Design review of the part built by this model. Coordinates are the model's own, in mm. Face numbers are marked on the shaded views. A direction names the side the tool comes from. Coordinates: 2 decimals unless noted, no trailing zeros. Loops run counter-clockwise (first coordinate to the right, second up) from the corner with the lowest first, then second, coordinate; pieces in that order, holes last. Notation, with made-up numbers: M 14.5,15.25 L 67.5,15.25 A12 ccw 67.5,19.25 Z; hole C -23,57 d6. An arc over 180 degrees is marked long. Put each result on its own line as item: value. Start each with the question number.
(1) For probe 1 along X at (y, z) = (35.25, 2.75); probe 2 along X at (y, z) = (-35.25, 5.75), list the stretches that pass through material, from the lowest coordinate up. Write a range as [from, to].
(2) Take a section at C-C, the plane y = 0. Give the boundary of the cut face in (x, z).
(3) For the marked faces 4, 5 and 6, list the 3-axis set-ups (+Z, -Z, +X, -X, +Y, -Y) from which the entire face can be reached by the end or side of a thin tool; tool diameter is ignored.
(4) Take a section at B-B, the plane x = -1. Give the boundary of the cut face in (y, z), then the cut area to 3 significant figures.
(5) Clearance check with a flat-ended pin moving along its axis: pin 1 (3.5 mm diameter, centred on x = -6.5, y = 31, fed in from +Z). State where the tip first meets the part, or that it passes through.
(6) Take a section at D-D, the plane y = 35.25. Give the boundary of the cut face in (x, z), then the cut area to 3 significant figures.
(7) The part is to be moulded in two halves that separate along X. For the marked faces 1, 2 and 3, say which applies: +X half, -X half, draft (parallel to the pull), parting line (faces both ways), or undercut.
(8) Take a section at A-A, the plane y = 14.5. Give the boundary of the cut face in (x, z).
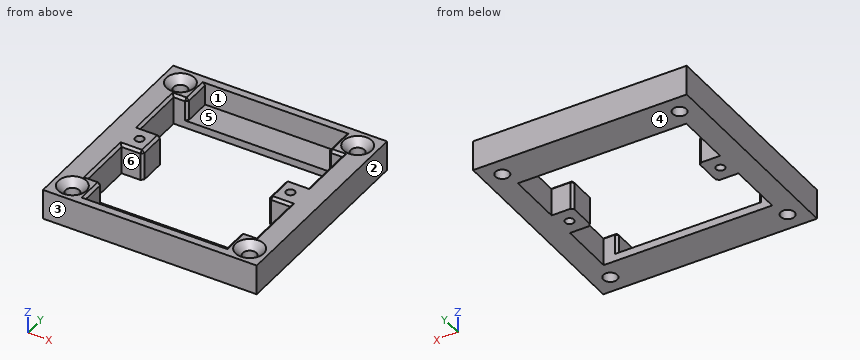
```python
from build123d import *

# Parameters (mm, degrees)
F0_W           = 9
F0_H           = 12
F0_W_2         = 8.5
F1_DEPTH       = 12
F3_D           = 3.5
F4_D           = 5.5
F4_CSINK_D     = 11.2
F4_CSINK_ANGLE = 90
F5_W           = 56
F5_H           = 11.5
F6_DEPTH       = 9
F7_SIZE        = 1


with BuildPart() as f1:
    # F0 (on Top) → F1 (new body)
    with BuildSketch(Plane.XY):
        Polygon((-42.5, -6), (-42.5, -42.5), (42.5, -42.5), (42.5, -6), (33.5, -6), (33.5, -28), (-33.5, -28), (-33.5, -6), align=None)
        Polygon((-42.5, 42.5), (-42.5, 6), (-33.5, 6), (-33.5, 28), (33.5, 28), (33.5, 6), (42.5, 6), (42.5, 42.5), align=None)
        with Locations((-38, 0)):
            Rectangle(F0_W, F0_H)
        with Locations((-29.25, 0)):
            Rectangle(F0_W_2, F0_H)
        with Locations((38, 0)):
            Rectangle(F0_W, F0_H)
        with Locations((29.25, 0)):
            Rectangle(F0_W_2, F0_H)
    extrude(amount=F1_DEPTH)

    # F3 (through all)
    with Locations(Plane.XY.offset(12)):
        with Locations((-30, 0), (30, 0)):
            Hole(F3_D / 2)

    # F4 (through all)
    with Locations(Plane.XY.offset(12)):
        with Locations((-35.25, 35.25), (35.25, 35.25), (35.25, -35.25), (-35.25, -35.25)):
            CounterSinkHole(F4_D / 2, F4_CSINK_D / 2, counter_sink_angle=F4_CSINK_ANGLE)

    # F5 (on face) → F6 (cut)
    with BuildSketch(Plane.XY.offset(12)):
        with Locations((0, -33.75)):
            Rectangle(F5_W, F5_H)
        with Locations((0, 33.75)):
            Rectangle(F5_W, F5_H)
    extrude(amount=-F6_DEPTH, mode=Mode.SUBTRACT)

    # F7
    f7_edges = [f1.edges().sort_by_distance(p)[0] for p in [
        (-30.75, 28, 12),
        (-33.5, 17, 12),
        (-29.25, 6, 12),
        (-25, 0, 12),
        (-29.25, -6, 12),
        (-33.5, -17, 12),
        (-30.75, -28, 12),
        (30.75, 28, 12),
        (33.5, 17, 12),
        (29.25, 6, 12),
        (25, 0, 12),
        (29.25, -6, 12),
        (33.5, -17, 12),
        (30.75, -28, 12),
        (-28, -28, 7.5),
        (28, -28, 7.5),
        (-28, 28, 7.5),
        (28, 28, 7.5),
        (-25, 6, 6),
        (-25, -6, 6),
        (25, 6, 6),
        (25, -6, 6),
        (-28, 33.75, 12),
        (28, 33.75, 12),
        (28, -33.75, 12),
        (-28, -33.75, 12),
    ]]
    chamfer(f7_edges, length=F7_SIZE)


solid = f1.part
```
Computed values:
1. probe 1: x = [-42.5, -38], [-32.5, 32.5], [38, 42.5]
1. probe 2: x = [-42.5, -38], [-32.5, -28], [28, 32.5], [38, 42.5]
2. outline: M -42.5,0 L -31.75,0 L -31.75,12 L -42.5,12 Z; M -28.25,0 L -25,0 L -25,11 L -26,12 L -28.25,12 Z; M 25,0 L 28.25,0 L 28.25,12 L 26,12 L 25,11 Z; M 31.75,0 L 42.5,0 L 42.5,12 L 31.75,12 Z
3. face 4: -Z, +X, -X, +Y, -Y
3. face 5: +Z
3. face 6: +Z, -Z
4. outline: M -42.5,0 L -28,0 L -28,3 L -39.5,3 L -39.5,12 L -42.5,12 Z; M 28,0 L 42.5,0 L 42.5,12 L 39.5,12 L 39.5,3 L 28,3 Z
4. area: 141 mm^2
5. pin 1: stops at z = 3
6. outline: M -42.5,0 L -38,0 L -38,9.15 L -40.85,12 L -42.5,12 Z; M -32.5,0 L 32.5,0 L 32.5,9.15 L 29.65,12 L 29,12 L 28,11 L 28,3 L -28,3 L -28,11 L -29,12 L -29.65,12 L -32.5,9.15 Z; M 38,0 L 42.5,0 L 42.5,12 L 40.85,12 L 38,9.15 Z
6. area: 367 mm^2
7. face 1: undercut
7. face 2: +X half
7. face 3: draft
8. outline: M -42.5,0 L -33.5,0 L -33.5,11 L -34.5,12 L -42.5,12 Z; M 33.5,0 L 42.5,0 L 42.5,12 L 34.5,12 L 33.5,11 Z
